from build123d import *

# Parameters (mm, degrees)
F0_W     = 261.9375
F0_H     = 61.9125
F1_DEPTH = 42.8625
F2_R     = 5.55625
F2_W     = 34.925
F2_H     = 19.05
F2_W_2   = 222.25
F2_H_2   = 15.875
F3_DEPTH = 39.6875
F4_R     = 13.49375
F5_DEPTH = 15.875


# Not quite as in the source:
# - a feature of the source that left no trace in its solid (it failed there, or was rolled back) is left out


with BuildPart() as f1:
    # F0 (on Top) → F1 (new body)
    with BuildSketch(Plane.XY):
        with Locations((130.96875, 30.95625)):
            Rectangle(F0_W, F0_H)
    extrude(amount=F1_DEPTH)

    # F2 (on face) → F3 (cut, through all)
    with BuildSketch(Plane.XY.offset(42.8625)):
        with Locations((16.66875, 53.18125)):
            Circle(F2_R)
        with Locations((48.3302816571, 49.2125)):
            Rectangle(F2_W, F2_H)
        with Locations((147.6375, 11.1125)):
            Rectangle(F2_W_2, F2_H_2)
    extrude(amount=-F3_DEPTH, mode=Mode.SUBTRACT)

    # F4 (on face) → F5 (cut)
    with BuildSketch(Plane.XY.offset(42.8625)):
        with Locations((16.66875, 30.95625)):
            Circle(F4_R)
        with BuildLine():
            Line((3.175, 19.05), (3.175, 3.175))
            Line((3.175, 3.175), (33.3375, 3.175))
            Line((33.3375, 3.175), (33.3375, 19.05))
            Line((33.3375, 19.05), (28.3344449, 19.05))
            ThreePointArc((28.3344449, 19.05), (16.66875, 14.2875), (5.0030551, 19.05))
            Line((5.0030551, 19.05), (3.175, 19.05))
        make_face()
    extrude(amount=-F5_DEPTH, mode=Mode.SUBTRACT)


solid = f1.part
Work out the finished part from the listing and answer in its coordinate system (mm). A direction names the side the tool comes from. Give positions to 0.01 mm unless a question says otherwise; leave off trailing zeros. Order: outer loops, then holes, each group sorted by start corner. A loop starts at its lowest first (then second) coordinate and runs counter-clockwise, first axis right, second up. Notation, with made-up numbers: (34.25, 18) - (91.25, 18) arc R24 ccw to (91.25, 50) - close; hole circle Ø11 at (24, 61). An arc over 180 degrees is marked (long way). Answer as CSV lines item,"result". Start each with the question number.
Q1. The part is cut by section C-C (z = 37.5). Give the number of separate pieces and of enclosed holes in the cut face, then the cut area to 3 significant figures.
Q2. Given pin 1 Ø15 at (x, y) = (46.5, 47.5) entering from +Z (3 decimals), flat-ended and moving along its own axis, determine where the tip first touches the part or whether it passes through.
Q3. Find the intervals of material crossed by L1, parallel to X at y = 53, z = 11; L2, parallel to X at y = 9.5, z = 34.5 (1 decimal); L3, parallel to X at y = 17, z = 5.5, in increasing order. Write a range as [from, to].
Q4. The part is cut by section A-A (y = 11). Write down the section's boundary in (x, z) (1 decimal), then the cut area to 3 significant figures.
Q5. The mould has two halves that part along X. Classify faces 1 (the face through (129, 31, 0)), 2 (the face through (261.938, 31, 21)), 3 (the face through (16.85, 14.29, 35.04)): +X half, -X half, draft (parallel to the pull), parting line (faces both ways), or undercut.
Q6. For faces 4 (the face through (129, 38, 42.862)), 5 (the face through (17, 53, 3.175)), determine the directions among +Z, -Z, +X, -X, +Y, -Y from which every point of the face is accessible in a straight line to the end or side of a thin tool.
Check result:
1,separate pieces,"1"
1,enclosed holes,"5"
1,area,"11,000 mm²"
2,pin 1,"stops at z = 3.175"
3,L1,"x = [0, 11.12], [22.22, 30.87], [65.79, 261.94]"
3,L2,"x = [0, 3.2], [33.3, 36.5], [258.8, 261.9]"
3,L3,"x = [0, 36.51], [258.76, 261.94]"
4,outline,"(0, 0) - (261.9, 0) - (261.9, 42.9) - (258.8, 42.9) - (258.8, 3.2) - (36.5, 3.2) - (36.5, 42.9) - (33.3, 42.9) - (33.3, 27) - (3.2, 27) - (3.2, 42.9) - (0, 42.9) - close"
4,area,"1,930 mm²"
5,face 1,"draft"
5,face 2,"+X half"
5,face 3,"undercut"
6,face 4,"+Z, +X, -X, +Y, -Y"
6,face 5,"+Z"
